Design review of the part built by this model. Coordinates are the model's own, in mm. A direction names the side the tool comes from. Coordinates: 2 decimals unless noted, no trailing zeros. Order: outer loops, then holes, each group sorted by start corner. A loop starts at its lowest first (then second) coordinate and runs counter-clockwise, first axis right, second up. Notation, with made-up numbers: (37.25, 84.25) -> (59.25, 84.25) arc R19 ccw to (59.25, 111.25) -> close; hole circle Ø8 at (38, 3). An arc over 180 degrees is marked (long way). Write item = value, one per line.
```python
from build123d import *

# Parameters (mm, degrees)
F1_DEPTH = 50.8
F3_DEPTH = 12.701
F4_W     = 19.05
F4_H     = 14.675198
F5_DEPTH = 19.05
F7_DEPTH = 30.798499


with BuildPart() as f1:
    # F0 (on Front) → F1 (new body)
    with BuildSketch(Plane.XZ):
        Polygon((-42.055184, 37.533606), (-54.755184, 37.533606), (-54.755184, 5.783606), (-23.005184, 5.783606), (-23.005184, 18.483606), (-42.055184, 18.483606), align=None)
    extrude(amount=F1_DEPTH)

    # F2 (on face) → F3 (cut, through all)
    with BuildSketch(Plane.YZ.offset(-42.055184)):
        Polygon((0, 37.533606), (-12.7, 37.533606), (0, 18.483606), align=None)
    extrude(amount=-F3_DEPTH, mode=Mode.SUBTRACT)

    # F4 (on face) → F5 (join)
    with BuildSketch(Plane.XY.offset(18.483606)):
        with Locations((-32.530184, -27.3401)):
            Rectangle(F4_W, F4_H)
    extrude(amount=F5_DEPTH)

    # F6 (on face) → F7 (cut, through all)
    with BuildSketch(Plane(origin=(0, -20.002501, 0), x_dir=(-1, 0, 0), z_dir=(0, 1, 0))):
        Polygon((23.005184, 18.483606), (42.055184, 37.533606), (23.005184, 37.533606), align=None)
    extrude(amount=-F7_DEPTH, mode=Mode.SUBTRACT)


solid = f1.part
```
(1) We need section C-C (z = 26). Write out the cut boundary in (x, y).
Report:
outline = (-54.76, -50.8) -> (-42.06, -50.8) -> (-42.06, -34.68) -> (-30.52, -34.68) -> (-30.52, -20) -> (-42.06, -20) -> (-42.06, -5.01) -> (-54.76, -5.01) -> close
(2) For L1, parallel to X at y = -18, z = 28.5; L2, parallel to Y at x = -31, z = 20; L3, parallel to Z at x = -26.5, y = -5, list the stretches that pass through material, from the lowest coordinate up.
Report:
L1 = -54.76 to -42.06
L2 = -34.68 to -20
L3 = 5.78 to 18.48
(3) Insertion check: pin 1 (4 mm diameter, centred on x = -31, z = 24.5, fed in from -Y); pin 2 (15 mm diameter, centred on y = -9.5, z = 29.5, fed in from +X); pin 3 (5 mm diameter, centred on y = -18, z = 24, fed in from +X). Each pin has a flat end and moves straight along its axis. Give the tip position at first contact, or say it passes through.
Report:
pin_1 = -34.68
pin_2 = -42.06
pin_3 = -27.02
(4) We need section D-D (x = -44.5). Write out the cut boundary in (y, z), and give its area (3 significant figures).
Report:
outline = (-50.8, 5.78) -> (0, 5.78) -> (0, 18.48) -> (-12.7, 37.53) -> (-50.8, 37.53) -> close
area = 1,490 mm²
(5) For faces 4 (the flat face through (-54.755, -25, 22)), 5 (the flat face through (-32, -10, 18.484)), 6 (the flat face through (-42.055, -43, 28)), list the 3-axis set-ups (+Z, -Z, +X, -X, +Y, -Y) from which the entire face can be reached by the end or side of a thin tool; tool diameter is ignored.
Report:
face_4 = +Z, -Z, -X, +Y, -Y
face_5 = +Z, +X, +Y
face_6 = +Z, +X, -Y
(6) We need section A-A (y = -14.5). Write out the cut boundary in (x, z), and give its area (3 significant figures).
Report:
outline = (-54.76, 5.78) -> (-23.01, 5.78) -> (-23.01, 18.48) -> (-42.06, 18.48) -> (-42.06, 37.53) -> (-54.76, 37.53) -> close
area = 645 mm²
(7) The part is to be moulded in two halves that separate along Z. For faces 1 (the flat face through (-43, -50.8, 18)), 2 (the flat face through (-48, -31, 37.534)), 3 (the flat face through (-39, -25, 5.784)), say which applies: released by +Z, released by -Z, zero draft, split by the parting line, or undercut.
Report:
face_1 = zero draft
face_2 = released by +Z
face_3 = released by -Z
(8) We need section B-B (x = -27.5). Write out the cut boundary in (y, z).
Report:
outline = (-50.8, 5.78) -> (0, 5.78) -> (0, 18.48) -> (-20, 18.48) -> (-20, 22.98) -> (-34.68, 22.98) -> (-34.68, 18.48) -> (-50.8, 18.48) -> close
